```python
from build123d import *

# Parameters (mm, degrees)
SKETCH1_R                    = 50
BOSS_EXTRUDE1_DEPTH          = 9
SKETCH2_R                    = 2.4
BOSS_EXTRUDE2_DEPTH          = 7
CHAMFER1_SIZE                = 1
CIRPATTERN1_COUNT            = 12
CHAMFER1_OF_CIRPATTERN1_SIZE = 1
SKETCH3_R                    = 32.15
CUT_EXTRUDE1_DEPTH           = 4
SKETCH4_R                    = 12
CUT_EXTRUDE2_DEPTH           = 10
CHAMFER2_SIZE                = 0.6
SKETCH5_R                    = 29.3
SKETCH5_R_2                  = 18.7
CUT_EXTRUDE3_DEPTH           = 2
CHAMFER3_SIZE                = 0.2
CHAMFER4_SIZE                = 3
CHAMFER5_SIZE                = 1
CHAMFER6_SIZE                = 0.6


with BuildPart() as part:
    # Sketch1 → Boss-Extrude1 (new body)
    with BuildSketch(Plane.XY):
        Circle(SKETCH1_R)
    extrude(amount=-BOSS_EXTRUDE1_DEPTH)

    # Sketch2 → Boss-Extrude2 (add)
    with BuildSketch(Plane.XY):
        with Locations((45, 0)):
            Circle(SKETCH2_R)
    boss_extrude2 = extrude(amount=BOSS_EXTRUDE2_DEPTH)

    # Chamfer1
    chamfer1_edges = [part.edges().sort_by_distance(p)[0] for p in [
        (42.6, 0, 7),
    ]]
    chamfer(chamfer1_edges, length=CHAMFER1_SIZE)

    # CirPattern1: Boss-Extrude2 ×12 about axis
    cirpattern1_axis = Axis((0, 0, 0), (0, 0, 1))
    for i in range(1, CIRPATTERN1_COUNT):
        add(boss_extrude2.rotate(cirpattern1_axis, i * 360 / CIRPATTERN1_COUNT))

    # Chamfer1 of CirPattern1
    chamfer1_of_cirpattern1_edges = [part.edges().sort_by_distance(p)[0] for p in [
        (36.892682201, 21.3, 7),
        (21.3, 36.892682201, 7),
        (0, 42.6, 7),
        (-21.3, 36.892682201, 7),
        (-36.892682201, 21.3, 7),
        (-42.6, 0, 7),
        (-36.892682201, -21.3, 7),
        (-21.3, -36.892682201, 7),
        (0, -42.6, 7),
        (21.3, -36.892682201, 7),
        (36.892682201, -21.3, 7),
    ]]
    chamfer(chamfer1_of_cirpattern1_edges, length=CHAMFER1_OF_CIRPATTERN1_SIZE)

    # Sketch3 → Cut-Extrude1 (cut)
    with BuildSketch(Plane.XY):
        Circle(SKETCH3_R)
    extrude(amount=-CUT_EXTRUDE1_DEPTH, mode=Mode.SUBTRACT)

    # Sketch4 → Cut-Extrude2 (cut, through all)
    with BuildSketch(Plane.XY):
        Circle(SKETCH4_R)
    extrude(amount=-CUT_EXTRUDE2_DEPTH, mode=Mode.SUBTRACT)

    # Chamfer2
    chamfer2_edges = [part.edges().sort_by_distance(p)[0] for p in [
        (-32.15, 0, 0),
    ]]
    chamfer(chamfer2_edges, length=CHAMFER2_SIZE)

    # Sketch5 → Cut-Extrude3 (cut)
    with BuildSketch(Plane.XY.offset(-4)):
        Circle(SKETCH5_R)
        Circle(SKETCH5_R_2, mode=Mode.SUBTRACT)
    extrude(amount=-CUT_EXTRUDE3_DEPTH, mode=Mode.SUBTRACT)

    # Chamfer3
    chamfer3_edges = [part.edges().sort_by_distance(p)[0] for p in [
        (-29.3, 0, -4),
        (-18.7, 0, -4),
    ]]
    chamfer(chamfer3_edges, length=CHAMFER3_SIZE)

    # Chamfer4
    chamfer4_edges = [part.edges().sort_by_distance(p)[0] for p in [
        (-50, 0, -9),
    ]]
    chamfer(chamfer4_edges, length=CHAMFER4_SIZE)

    # Chamfer5
    chamfer5_edges = [part.edges().sort_by_distance(p)[0] for p in [
        (-12, 0, -9),
    ]]
    chamfer(chamfer5_edges, length=CHAMFER5_SIZE)

    # Chamfer6
    chamfer6_edges = [part.edges().sort_by_distance(p)[0] for p in [
        (-12, 0, -4),
    ]]
    chamfer(chamfer6_edges, length=CHAMFER6_SIZE)


solid = part.part
```
CAD build for the part. Positions are in the model's coordinates, mm. A direction names the side the tool comes from. Round coordinates to 2 decimals unless told otherwise and drop trailing zeros.
Item 1: Band-saw the part on A-A on z = 3. Give the number of separate pieces and of enclosed holes in the cut face, then the cut area to 3 significant figures.
Filled in:
separate pieces: 12
enclosed holes: 0
area: 217 mm2
Item 2: Drill centre lines: L1, parallel to Y at x = 0, z = -4.5; L2, parallel to Y at x = 0, z = -3; L3, parallel to X at y = -6.5, z = -5. Where is each one in solid material? Low to high.
Filled in:
L1: y = -50 to -29.3, -18.7 to -12.1, 12.1 to 18.7, 29.3 to 50
L2: y = -50 to -32.15, 32.15 to 50
L3: x = -49.58 to -28.57, -17.53 to -10.09, 10.09 to 17.53, 28.57 to 49.58
Item 3: Mould opens along Y. For faces 1 (the flat face through (-45, 0, 7)), 2 (the flat face through (10, -33, 0)), 3 (the cylindrical face through (42.602, 0.106, 2.958)) say: released by +Y, released by -Y, zero draft, split by the parting line, or undercut.
Filled in:
face 1: zero draft
face 2: undercut
face 3: split by the parting line
Item 4: Drop flat-ended pins along their axis: pin 1 Ø5 at (x, z) = (-9, 4.5) entering from -Y; pin 2 Ø11 at (x, y) = (7, -5.5) entering from +Z; pin 3 Ø1 at (x, y) = (34.5, -15.5) entering from +Z; pin 4 Ø4 at (y, z) = (-38, 3.5) entering from -X. Give the stop position or say it passes through.
Filled in:
pin 1: passes through
pin 2: stops at z = -4
pin 3: stops at z = 0
pin 4: stops at x = -24.9
Item 5: Tool access for faces 4 (the flat face through (39, -22, 7)), 5 (the cylindrical face through (-36.63, -23.02, 2.96)): list every direction of +Z, -Z, +X, -X, +Y, -Y with a clear straight run to the whole face (end or side of a thin tool).
Filled in:
face 4: +Z, +X, -X, +Y, -Y
face 5: +Z
